Work out the finished part from the listing and answer in its coordinate system (mm). Coordinates: 2 decimals unless noted, no trailing zeros. Order: outer loops, then holes, each group sorted by start corner. A loop starts at its lowest first (then second) coordinate and runs counter-clockwise, first axis right, second up. Notation, with made-up numbers: M -9,86 L 39,86 A21 ccw 39,91 Z; hole C 64,64.5 d10. An arc over 180 degrees is marked long. Answer in a Markdown table with one row per item. Add a question column.
Item 1: The part is cut by section B-B (z = 1.75). Write down the section's boundary in (x, y).
Item 2: Flat-ended cylindrical pins translate along their axes: pin 1 Ø1 at (x, y) = (-15, -30.5) entering from -Z; pin 2 Ø3 at (y, z) = (17, 3.5) entering from -X; pin 3 Ø23 at (x, y) = (-21.65, 12.5) entering from +Z. Find the tip coordinate at first contact, or state that the pin passes through.
Item 3: The mould has two halves that part along X. Classify faces 1 (the face through (11, -4, 0)), 2 (the face through (34.9, 19.53, 2.96)): released by +X, released by -X, zero draft, split by the parting line, or undercut.
Item 4: The part is cut by section A-A (y = -25). Write down the section's boundary in (x, z), then the cut area to 3 significant figures.
Item 5: Consider line 1 (Y direction, x = -2, z = 0.35); line 2 (Y direction, x = -10, z = 0.9); line 3 (X direction, y = 8.5, z = 0.8). Determine where each line is inside the solid, lowest interval first. Write a range as from..to.
Item 6: The part is cut by section C-C (x = -23). Write down the section's boundary in (y, z).
Item 7: The part is cut by section D-D (y = 12.5). Write down the section's boundary in (x, z), then the cut area to 3 significant figures.
from build123d import *

# Parameters (mm, degrees)
F0_R     = 9.95
F1_DEPTH = 6


with BuildPart() as f1:
    # F0 (on Top) → F1 (new body)
    with BuildSketch(Plane.XY):
        with BuildLine():
            ThreePointArc((-12.990381, -7.5), (-10.930703, -10.272279), (-8.291562, -12.5))
            ThreePointArc((-8.291562, -12.5), (0, -40), (8.291562, -12.5))
            ThreePointArc((8.291562, -12.5), (10.930703, -10.272279), (12.990381, -7.5))
            ThreePointArc((12.990381, -7.5), (14.361407, -4.330127), (14.971099, -0.930703))
            ThreePointArc((14.971099, -0.930703), (34.641016, 20), (6.679537, 13.430703))
            ThreePointArc((6.679537, 13.430703), (3.430703, 14.602406), (0, 15))
            ThreePointArc((0, 15), (-3.430703, 14.602406), (-6.679537, 13.430703))
            ThreePointArc((-6.679537, 13.430703), (-34.641016, 20), (-14.971099, -0.930703))
            ThreePointArc((-14.971099, -0.930703), (-14.361407, -4.330127), (-12.990381, -7.5))
        make_face()
        with Locations((0, -25)):
            Circle(F0_R, mode=Mode.SUBTRACT)
        with BuildLine():
            ThreePointArc((9.526279, -5.5), (0, -11), (-9.526279, -5.5))
            ThreePointArc((-9.526279, -5.5), (-9.526279, 5.5), (0, 11))
            ThreePointArc((0, 11), (9.526279, 5.5), (9.526279, -5.5))
        make_face(mode=Mode.SUBTRACT)
        with Locations((-21.650635, 12.5)):
            Circle(F0_R, mode=Mode.SUBTRACT)
        with Locations((21.650635, 12.5)):
            Circle(F0_R, mode=Mode.SUBTRACT)
    extrude(amount=F1_DEPTH)


solid = f1.part
Reply:
| question | item | result |
|---|---|---|
| 1 | outline | M -14.97,-0.93 A15 ccw -12.99,-7.5 A15 ccw -8.29,-12.5 A15 ccw long 8.29,-12.5 A15 ccw 12.99,-7.5 A15 ccw 14.97,-0.93 A15 ccw long 6.68,13.43 A15 ccw 0,15 A15 ccw -6.68,13.43 A15 ccw long Z; hole C -21.65,12.5 d19.9; hole C 0,0 d22; hole C 0,-25 d19.9; hole C 21.65,12.5 d19.9 |
| 2 | pin 1 | passes through |
| 2 | pin 2 | stops at x = -36.35 |
| 2 | pin 3 | stops at z = 6 |
| 3 | face 1 | zero draft |
| 3 | face 2 | undercut |
| 4 | outline | M -15,0 L -9.95,0 L -9.95,6 L -15,6 Z; M 9.95,0 L 15,0 L 15,6 L 9.95,6 Z |
| 4 | area | 60.6 mm2 |
| 5 | line 1 | y = -39.87..-34.75, -15.25..-10.82, 10.82..14.87 |
| 5 | line 2 | y = -36.18..-13.82, -11.18..-4.58, 4.58..21.95 |
| 5 | line 3 | x = -36.11..-30.76, -12.54..-6.98, 6.98..12.54, 30.76..36.11 |
| 6 | outline | M -2.44,0 L 2.64,0 L 2.64,6 L -2.44,6 Z; M 22.36,0 L 27.44,0 L 27.44,6 L 22.36,6 Z |
| 7 | outline | M -36.65,0 L -31.6,0 L -31.6,6 L -36.65,6 Z; M -11.7,0 L 11.7,0 L 11.7,6 L -11.7,6 Z; M 31.6,0 L 36.65,0 L 36.65,6 L 31.6,6 Z |
| 7 | area | 201 mm2 |
